Autodesk Inventor part; units mm, degrees
ref_plane "Work Plane1" through (0, -10, 0) normal (0, 1, 0) x (-1, 0, 0)
ref_plane "Work Plane2" through (10, -25, 10) normal (-0.7071, 0, 0.7071) x (0, 1, 0)
ref_plane "YZ Plane" through (0, 0, 0) normal (1, 0, 0) x (0, 1, 0)
sketch "Sketch1" plane through (0, 0, 0) normal (0, 0, 1) x (1, 0, 0)
  line L0 (-10, 25) -> (10, 25)
  line L1 (10, 25) -> (10, -25)
  line L2 (10, -25) -> (-10, -25)
  line L3 (-10, -25) -> (-10, 25)
  circle A0 centre (0, 18) radius 2.5
  circle A1 centre (0, -18) radius 2.5
  point P0 (0, 0)
  point P1 (-10, 0)
  point P2 (0, 25)
  dimension "d0" = 20
  dimension "d1" = 50
  dimension "d2" = 5
  dimension "d3" = 7
  dimension "d4" = 7
extrude "Extrusion1" add sketch "Sketch1" along normal blind 10
ref_plane "Work Plane1" through (0, -10, 0) normal (0, 1, 0) x (-1, 0, 0)
ref_plane "Work Plane2" through (10, -25, 10) normal (-0.7071, 0, 0.7071) x (0, 1, 0)
sketch "Sketch7" plane through (10, -25, 10) normal (0, 0, 1) x (0, 1, 0)
  line L0 (50, 0) -> (0, 0)
  circle A0 centre (25, 10) radius 10
  line L1 (50, 20) -> (0, 20)
  circle A1 centre (43, 10) radius 2.5
  circle A2 centre (7, 10) radius 2.5
  line L2 (0, 20) -> (50, 20)
  line L3 (50, 20) -> (50, 0)
  line L4 (0, 0) -> (0, 20)
  point P0 (25, 10)
  point P1 (25, 20)
  dimension "d28" = 20
  dimension "d29" = 10
extrude "Extrusion6" add sketch "Sketch7" along normal blind 30 contours A0
sketch "Sketch8" plane through (0, 0, 0) normal (0, 1, 0) x (-1, 0, 0)
  circle A0 centre (0, 40) radius 10
  line L0 (-10, 10) -> (-10, 40)
  line L1 (-10, 40) -> (10, 40)
  line L2 (10, 40) -> (10, 10)
  line L3 (10, 10) -> (10, 0)
  line L4 (10, 0) -> (-10, 0)
  line L5 (-10, 0) -> (-10, 10)
  point P0 (0, 0)
  point P1 (25.3553, 31.2132)
  point P2 (-10, 3.7868)
  dimension "d47" = 20
extrude "Extrusion7" add sketch "Sketch8" along normal mid plane 20 contours L1 A0 | A0 L1
sketch "Sketch9" plane through (0, 10, 40) normal (0, 1, 0) x (1, 0, 0)
  circle A0 centre (0, 0) radius 4
  circle A1 centre (0, 0) radius 10
  point P0 (0, 40)
  point P1 (-3.2583, 9.4543)
  point P2 (3.2583, 9.4543)
  point P3 (-2.6421, 9.6447)
  point P4 (2.6421, 9.6447)
  point P5 (0, 10)
  point P6 (0, 10)
  dimension "d35" = 8
extrude "Extrusion8" cut sketch "Sketch9" against normal through all contours A0
equation "\"d4\" = d3"
properties part number "10-06-008"
Source: CAD feature listing. Evaluate the final solid. Frame: model axes, mm. A direction names the side the tool comes from. Round coordinates to 2 decimals unless told otherwise and drop trailing zeros. Write each loop counter-clockwise with the first axis right and the second up, starting at its lowest first coordinate (ties: lowest second). Pieces come first, ordered by that corner, then holes. Notation, with made-up numbers: (-28.75, 0) - (11.25, 0) arc R28 cw to (11.25, 32) - close; hole circle Ø2 at (-20, 44.5). An arc over 180 degrees is marked (long way). Use CSV: the item, a comma, the result in double quotes. Start each with the question number.
(1) First-contact query: pin 1 Ø1.5 at (y, z) = (8.5, 38) entering from +X; pin 2 Ø10 at (x, z) = (-1.5, 42) entering from -Y; pin 3 Ø6 at (y, z) = (-3, 43.5) entering from +X. Flat tips, straight axial feed; report the tip coordinate or a pass-through.
(2) Cut plane D-D, the plane x = -8.25. Return loops of the section in (y, z).
(3) Mould query, pull axis X, two halves, no side actions, for faces 1 (the face through (2.385, 17.249, 4.93)), 2 (the face through (0, 15, 10)), 3 (the face through (0, -10, 21)), 4 (the face through (-0.33, -20.48, 4.93)). Classes: pulls with the +X half, pulls with the -X half, needs draft (parallel to the pull), parting line crosses it, or undercut.
(4) Cut plane C-C, the plane z = 7.5. Return loops of the section in (x, y), and give its area (3 significant figures).
(5) Cut plane B-B, the plane y = 8. Return loops of the section in (x, z), and give its area (3 significant figures).
(6) Cut plane A-A, the plane y = 18. Return loops of the section in (x, z).
(7) Set-up query: faces 5 (the face through (0.1, 10, 35.7)), 6 (the face through (0.1, -10, 35.7)), 7 (the face through (0, 25, 5)). Return all of +Z, -Z, +X, -X, +Y, -Y with unobstructed straight access to the full face (end or side cutting, diameter ignored); none if empty.
(8) Material intervals for probe 1 along Y at (x, z) = (0, 6.5); probe 2 along X at (y, z) = (4, 40); probe 3 along Z at (x, y) = (0, 1), sorted ascending. Write a range as [from, to].
Geometry says:
1,pin 1,"x = 9.92"
1,pin 2,"y = -10"
1,pin 3,"x = 9.99"
2,outline,"(-25, 0) - (25, 0) - (25, 10) - (5.65, 10) - (5.65, 34.35) - (10, 34.35) - (10, 45.65) - (-10, 45.65) - (-10, 34.35) - (-5.65, 34.35) - (-5.65, 10) - (-25, 10) - close"
3,face 1,"undercut"
3,face 2,"needs draft"
3,face 3,"parting line crosses it"
3,face 4,"undercut"
4,outline,"(-10, -25) - (10, -25) - (10, 25) - (-10, 25) - close; hole circle Ø5 at (0, -18); hole circle Ø5 at (0, 18)"
4,area,"961 mm²"
5,outline,"(-10, 0) - (10, 0) - (10, 10) - (6, 10) - (6, 32) arc R10 ccw (long way) to (-6, 32) - (-6, 10) - (-10, 10) - close; hole circle Ø8 at (0, 40)"
5,area,"712 mm²"
6,outline,"(-10, 0) - (-2.5, 0) - (-2.5, 10) - (-10, 10) - close; (2.5, 0) - (10, 0) - (10, 10) - (2.5, 10) - close"
7,face 5,"+Z, +X, -X, +Y"
7,face 6,"+Z, +X, -X, -Y"
7,face 7,"+Z, -Z, +X, -X, +Y"
8,probe 1,"[-25, -20.5], [-15.5, 15.5], [20.5, 25]"
8,probe 2,"[-10, -4], [4, 10]"
8,probe 3,"[0, 36], [44, 50]"
